Geometry: final body of the model. Coordinates: model frame, mm. Coordinates: 2 decimals unless noted, no trailing zeros. Loops run counter-clockwise (first coordinate to the right, second up) from the corner with the lowest first, then second, coordinate; pieces in that order, holes last. Notation, with made-up numbers: (-3, 78.25) - (11, 78.25) arc R11 cw to (11, 85.25) - close; hole circle Ø3 at (-9.5, 61.25). An arc over 180 degrees is marked (long way). Write each question's results on one line, items separated by ' | '. Start each with the question number.
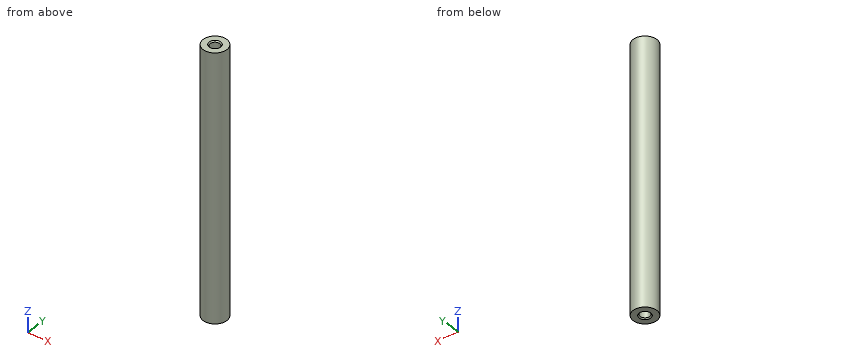
from build123d import *

# Parameters (mm, degrees)
ESBO_O1_R                           = 4.1
RESSALTO_EXTRUS_O1_DEPTH            = 91
FURO_ROSCADO_DE_M4X0_71_D           = 3.3
FURO_ROSCADO_DE_M4X0_71_DEPTH       = 11.5
FURO_ROSCADO_DE_M4X0_71_CSINK_D     = 4.05
FURO_ROSCADO_DE_M4X0_71_CSINK_ANGLE = 90
FURO_ROSCADO_DE_M4X0_71_TIP         = 0.991420021
FURO_ROSCADO_DE_M4X0_72_D           = 3.3
FURO_ROSCADO_DE_M4X0_72_DEPTH       = 11.5
FURO_ROSCADO_DE_M4X0_72_CSINK_D     = 4.05
FURO_ROSCADO_DE_M4X0_72_CSINK_ANGLE = 90
FURO_ROSCADO_DE_M4X0_72_TIP         = 0.991420021


with BuildPart() as part:
    # Esboço1 → Ressalto-extrusão1 (new body)
    with BuildSketch(Plane.XY):
        with Locations((-29.071712183, 179.873872767)):
            Circle(ESBO_O1_R)
    extrude(amount=-RESSALTO_EXTRUS_O1_DEPTH)

    # Furo roscado de M4x0.71
    with Locations(Plane.XY):
        with Locations((-29.071712183, 179.873872767)):
            CounterSinkHole(FURO_ROSCADO_DE_M4X0_71_D / 2, FURO_ROSCADO_DE_M4X0_71_CSINK_D / 2, depth=FURO_ROSCADO_DE_M4X0_71_DEPTH, counter_sink_angle=FURO_ROSCADO_DE_M4X0_71_CSINK_ANGLE)
            with Locations((0, 0, -(FURO_ROSCADO_DE_M4X0_71_DEPTH + FURO_ROSCADO_DE_M4X0_71_TIP / 2))):  # 118° drill point
                Cone(0, FURO_ROSCADO_DE_M4X0_71_D / 2, FURO_ROSCADO_DE_M4X0_71_TIP, mode=Mode.SUBTRACT)

    # Furo roscado de M4x0.72
    with Locations(Plane(origin=(0, 0, -91), x_dir=(-1, 0, 0), z_dir=(0, 0, -1))):
        with Locations((29.071712183, 179.873872767)):
            CounterSinkHole(FURO_ROSCADO_DE_M4X0_72_D / 2, FURO_ROSCADO_DE_M4X0_72_CSINK_D / 2, depth=FURO_ROSCADO_DE_M4X0_72_DEPTH, counter_sink_angle=FURO_ROSCADO_DE_M4X0_72_CSINK_ANGLE)
            with Locations((0, 0, -(FURO_ROSCADO_DE_M4X0_72_DEPTH + FURO_ROSCADO_DE_M4X0_72_TIP / 2))):  # 118° drill point
                Cone(0, FURO_ROSCADO_DE_M4X0_72_D / 2, FURO_ROSCADO_DE_M4X0_72_TIP, mode=Mode.SUBTRACT)


solid = part.part
1) Section query C-C on z = -35. Output: boundary loops of the cut face in (x, y).
2) Section query A-A on z = -83. Output: boundary loops of the cut face in (x, y).
3) Pin query (flat end, axial travel): pin 1 Ø1.5 at (y, z) = (181, -21) entering from +X; pin 2 Ø2 at (x, y) = (-29.07, 179.87) entering from -Z; pin 3 Ø1.5 at (x, z) = (-28, -61) entering from -Y. Return the tip coordinate at first contact, or that it passes through.
4) Material intervals for line 1 (X direction, y = 179.25, z = -10); line 2 (Y direction, x = -25.5, z = -43); line 3 (X direction, y = 178.5, z = -35.5), sorted ascending. Write a range as [from, to].
5) Section query B-B on x = -32. Output: boundary loops of the cut face in (y, z).
Returned:
1) outline: circle Ø8.2 at (-29.07, 179.87)
2) outline: circle Ø8.2 at (-29.07, 179.87); hole circle Ø3.3 at (-29.07, 179.87)
3) pin 1: stops at x = -24.99 | pin 2: stops at z = -79.11 | pin 3: stops at y = 175.79
4) line 1: x = [-33.12, -30.6], [-27.54, -25.02] | line 2: y = [177.86, 181.89] | line 3: x = [-32.93, -25.21]
5) outline: (177, -91) - (182.74, -91) - (182.74, 0) - (177, 0) - close
